Autodesk Inventor part; units mm, degrees
ref_plane "YZ Plane" through (0, 0, 0) normal (1, 0, 0) x (0, 1, 0)
ref_plane "XZ Plane" through (0, 0, 0) normal (0, 1, 0) x (-1, 0, 0)
ref_plane "XY Plane" through (0, 0, 0) normal (0, 0, 1) x (1, 0, 0)
sketch "スケッチ1" plane through (0, 0, 0) normal (0, 0, 1) x (1, 0, 0)
  circle A0 centre (7.9111, 33.2072) radius 1.1
  circle A1 centre (8.9353, 38.2023) radius 1.1
  circle A2 centre (-7.0645, 38.2798) radius 1.1
  circle A3 centre (-7.0888, 33.2799) radius 1.1
  spline S0 degree 3 poles (-12.8646, 33.9313) (-12.8659, 33.8333) (-12.8476, 33.7285) (-12.7708, 33.5355) (-12.7123, 33.4473) (-12.5725, 33.3024) (-12.4805, 33.2392) (-12.2855, 33.1578) (-12.1826, 33.1393) (-11.9746, 33.1367) (-11.8589, 33.1621) (-11.6558, 33.2543) (-11.5682, 33.3207) (-11.4449, 33.4571) (-11.3945, 33.5329) (-11.3402, 33.6628) (-11.3255, 33.7089) (-11.3046, 33.8062) (-11.2984, 33.8576) (-11.2971, 33.9662) (-11.302, 34.0177) (-11.3205, 34.1156) (-11.334, 34.1619) (-11.3851, 34.2932) (-11.4336, 34.3702) (-11.5535, 34.5096) (-11.6394, 34.5782) (-11.8401, 34.6754) (-11.9552, 34.7036) (-12.1632, 34.7062) (-12.2665, 34.6902) (-12.4635, 34.6136) (-12.557, 34.5528) (-12.7004, 34.4113) (-12.7611, 34.3246) (-12.8426, 34.1336) (-12.8634, 34.0293) (-12.8646, 33.9313) knots 0 0 0 0 0.029408 0.029408 0.058816 0.058816 0.090592 0.090592 0.122368 0.122368 0.162647 0.162647 0.202927 0.202927 0.235498 0.235498 0.251784 0.251784 0.26807 0.26807 0.284355 0.284355 0.300641 0.300641 0.333213 0.333213 0.373492 0.373492 0.413772 0.413772 0.445548 0.445548 0.477323 0.477323 0.506731 0.506731 0.536139 0.536139 0.536139 0.536139
  circle A4 centre (-17.0808, 33.9834) radius 0.7835
  arc A5 (-11.6308, 33.2805) -> (-11.6151, 34.5514) centre (-12.0812, 33.9216) ccw construction
  circle A6 centre (-12.0812, 33.9216) radius 1.1
  circle A7 centre (-17.0808, 33.9834) radius 1.1
  circle A8 centre (8.9353, 38.2023) radius 2
  circle A9 centre (-7.0645, 38.2798) radius 2
  circle A10 centre (-7.0888, 33.2799) radius 2
  circle A11 centre (7.9111, 33.2072) radius 2
  circle A12 centre (-12.0812, 33.9216) radius 2
  circle A13 centre (-17.0808, 33.9834) radius 2
  line L0 (8.945, 40.2023) -> (-7.0548, 40.2798)
  line L1 (9.8703, 32.8055) -> (10.8945, 37.8006)
  line L2 (7.9014, 31.2072) -> (-7.0985, 31.2799)
  line L3 (-7.8529, 40.1179) -> (-17.8692, 35.8215)
  line L4 (-17.2213, 31.9884) -> (-7.2292, 31.2848)
  line L5 (6.9761, 38.604) -> (5.9518, 33.6089)
  line L6 (8.9353, 38.2023) -> (-7.0645, 38.2798)
  line L7 (-5.0888, 33.2702) -> (-5.0645, 38.2701)
  line L8 (-7.0888, 33.2799) -> (7.9111, 33.2072)
  point P0 (0, 0)
  point P1 (-12.8646, 33.9313)
  point P2 (6.9353, 38.212)
  point P3 (6.8957, 38.2122)
  point P4 (5.9111, 33.2169)
extrude "押し出し1" add sketch "スケッチ1" along normal blind 1.5 contours A8 | A8 L5 L6 A9 L0 | L1 A11 L5 L6 A8 | A8 L6 L5 | A9 | A11 | A9 L7 A10 L4 A13 L3 | L2 A10 L8 A11 | A13 | A10 | A12
fillet "フィレット1" radius 2 4 edges at (6.8957, 38.2122, 0.75) (5.9111, 33.2169, 0.75) (-5.0645, 38.2701, 0.75) (-5.0888, 33.2702, 0.75)
properties part number "ude_tunagi" material "アルミニウム 2014-T4"
Geometry: final body of the model. Coordinates: model frame, mm. A direction names the side the tool comes from. Round coordinates to 2 decimals unless told otherwise and drop trailing zeros. Order: outer loops, then holes, each group sorted by start corner. A loop starts at its lowest first (then second) coordinate and runs counter-clockwise, first axis right, second up. Notation, with made-up numbers: (52.5, -31.75) -> (64.5, -31.75) arc R32 ccw to (64.5, -3.75) -> close; hole circle Ø10 at (65, 64). An arc over 180 degrees is marked (long way). Put each result on its own line as item: value. Start each with the question number.
Q1. Pull-direction query (Y, two-part tool) for faces 3 (the flat face through (-4, 33, 1.5)), 4 (the cylindrical face through (6.01, 37.47, 0.76)), 5 (the flat face through (10.375, 35.268, 0.74)); classes: +Y half, -Y half, draft (parallel to the pull), parting line (faces both ways), or undercut.
Q2. Section A-A on x = 0. Return the cut outline in (y, z), and give its area (3 significant figures).
Q3. Section C-C on y = 38.75. Return the cut outline in (x, z).
Q4. Line query: probe 1 along Y at (x, z) = (-7, 0.5); probe 2 along X at (y, z) = (38.5, 0.1); probe 3 along X at (y, z) = (34.5, 0.8). Output: solid intervals per line, ascending.
Q5. Section D-D on x = -16.5. Return the cut outline in (y, z).
Q6. Section B-B on y = 37.5. Return the cut outline in (x, z).
Q7. First-contact query: pin 1 (1.8 mm diameter, centred on x = -7.06, y = 38.28, fed in from +Z). Flat tip, straight axial feed; report the tip coordinate or a pass-through.
Q8. Reachability of faces 1 (the cylindrical face through (-4.466, 37.697, 0.76)), 2 (the cylindrical face through (-19.046, 33.613, 0.74)) from +Z, -Z, +X, -X, +Y, -Y: full face, straight path, thin tool, end or side. Return the list, or none.
Ans:
1. face 3: draft
1. face 4: undercut
1. face 5: -Y half
2. outline: (31.25, 0) -> (33.25, 0) -> (33.25, 1.5) -> (31.25, 1.5) -> close; (38.25, 0) -> (40.25, 0) -> (40.25, 1.5) -> (38.25, 1.5) -> close
2. area: 6.00 mm2
3. outline: (-11.04, 0) -> (-8.06, 0) -> (-8.06, 1.5) -> (-11.04, 1.5) -> close; (-6.07, 0) -> (7.98, 0) -> (7.98, 1.5) -> (-6.07, 1.5) -> close; (9.89, 0) -> (10.86, 0) -> (10.86, 1.5) -> (9.89, 1.5) -> close
4. probe 1: y = 31.28 to 32.18, 34.38 to 37.18, 39.38 to 40.28
4. probe 2: x = -11.62 to -8.14, -5.99 to 7.88, 9.99 to 10.91
4. probe 3: x = -19.01 to -18.05, -16.11 to -13.02, -11.15 to -4.93, 6.11 to 10.22
5. outline: (31.94, 0) -> (33.05, 0) -> (33.05, 1.5) -> (31.94, 1.5) -> close; (34.92, 0) -> (36.41, 0) -> (36.41, 1.5) -> (34.92, 1.5) -> close
6. outline: (-13.96, 0) -> (-7.84, 0) -> (-7.84, 1.5) -> (-13.96, 1.5) -> close; (-6.29, 0) -> (-4.64, 0) -> (-4.64, 1.5) -> (-6.29, 1.5) -> close; (5.99, 0) -> (8.09, 0) -> (8.09, 1.5) -> (5.99, 1.5) -> close; (9.78, 0) -> (10.83, 0) -> (10.83, 1.5) -> (9.78, 1.5) -> close
7. pin 1: passes through
8. face 1: +Z, -Z
8. face 2: +Z, -Z, -X
